Design review of the part built by this model. Coordinates are the model's own, in mm. A direction names the side the tool comes from. Round coordinates to 2 decimals unless told otherwise and drop trailing zeros. Write each loop counter-clockwise with the first axis right and the second up, starting at its lowest first coordinate (ties: lowest second). Pieces come first, ordered by that corner, then holes. Notation, with made-up numbers: (-19.5, -24.75) -> (-14.5, -24.75) arc R25 ccw to (-14.5, 11.25) -> close; hole circle Ø9 at (-25.5, 69.5). An arc over 180 degrees is marked (long way). One line per question, with ' | ' between items. Start each with the question number.
1) For probe 1 along Z at (x, y) = (-24.5, -16); probe 2 along Y at (x, z) = (-1.5, 101); probe 3 along Y at (x, z) = (-5.5, 125.5), list the stretches that pass through material, from the lowest coordinate up.
2) Insertion check: pin 1 Ø3.5 at (y, z) = (24, -1) entering from -X; pin 2 Ø18.5 at (x, y) = (3, -16.5) entering from +Z; pin 3 Ø8 at (x, z) = (-14, 12) entering from +Y; pin 4 Ø1.5 at (x, z) = (12.5, 80) entering from -Y. Each pin has a flat end and moves straight along its axis. Give the tip position at first contact, or say it passes through.
3) Consider section A-A (y = 0). Give the boundary of the cut face in (x, z) (3 decimals), then the cut area to 3 significant figures.
4) For faces 4 (the flat face through (6, 47.625, 64)), 5 (the flat face through (14.617, -24, -2)), 6 (the flat face through (6, 41.207, 66)), list the 3-axis set-ups (+Z, -Z, +X, -X, +Y, -Y) from which the entire face can be reached by the end or side of a thin tool; tool diameter is ignored.
5) Consider section C-C (x = 8). Give the boundary of the cut face in (y, z) (3 decimals), then the cut area to 3 significant figures.
6) Mouldability with a two-part tool opening along Y and no side actions: class faces 1 (the flat face through (17.792, 24, -2)), 2 (the flat face through (20.955, -1, -2)), 3 (the cylindrical face through (16.16, -39.688, -1.628)) as +Y half, -Y half, draft (parallel to the pull), parting line (faces both ways), or undercut.
7) Consider section D-D (y = -31.5). Give the boundary of the cut face in (x, z) (3 decimals), then the cut area to 3 significant figures.
8) Consider section B-B (z = 67). Give the boundary of the cut face in (x, y) (3 decimals).
```python
from build123d import *

# Parameters (mm, degrees)
F1_DEPTH = 133.35
F2_W     = 11.43
F2_H     = 95.25
F3_DEPTH = 6.35
F4_W     = 3.175
F4_H     = 7.62
F5_DEPTH = 3.302


with BuildPart() as f1:
    # F0 (on Top) → F1 (new body)
    with BuildSketch(Plane.XY):
        with BuildLine():
            Line((11.43, 47.625), (0, 47.625))
            ThreePointArc((0, 47.625), (-47.625, 0), (0, -47.625))
            Line((0, -47.625), (11.43, -47.625))
            Line((11.43, -47.625), (11.43, -41.232052))
            Line((11.43, -41.232052), (0, -41.232052))
            Line((0, -41.232052), (0, -41.275))
            ThreePointArc((0, -41.275), (-41.275, 0), (0, 41.275))
            Line((0, 41.275), (0, 41.207306))
            Line((0, 41.207306), (11.43, 41.207306))
            Line((11.43, 41.207306), (11.43, 47.625))
        make_face()
    extrude(amount=F1_DEPTH)

    # F2 (on Top) → F3 (join)
    with BuildSketch(Plane.XY):
        with BuildLine():
            Line((0, -47.625), (0, 47.625))
            ThreePointArc((0, 47.625), (-47.625, 0), (0, -47.625))
        make_face()
        with Locations((5.715, 0)):
            Rectangle(F2_W, F2_H)
    extrude(amount=-F3_DEPTH)

    # F4 (on face) → F5 (join)
    with BuildSketch(Plane.XY):
        with BuildLine():
            ThreePointArc((20.955, 38.890978), (16.227114, 39.752791), (11.43, 40.04145))
            Line((11.43, 40.04145), (11.43, -39.96855))
            ThreePointArc((11.43, -39.96855), (16.227114, -39.679891), (20.955, -38.818079))
            Line((20.955, -38.818079), (20.955, 38.890978))
        make_face()
        with Locations((16.204277, -24.09355)):
            Rectangle(F4_W, F4_H, mode=Mode.SUBTRACT)
        with Locations((16.1925, 0.03645)):
            Rectangle(F4_W, F4_H, mode=Mode.SUBTRACT)
        with Locations((16.204277, 24.16645)):
            Rectangle(F4_W, F4_H, mode=Mode.SUBTRACT)
    extrude(amount=-F5_DEPTH)


solid = f1.part
```
From the geometry:
1) probe 1: z = -6.35 to 0 | probe 2: y = -47.6 to -41.25, 41.25 to 47.6 | probe 3: y = -47.31 to -40.91, 40.91 to 47.31
2) pin 1: stops at x = -42.11 | pin 2: stops at z = 0 | pin 3: stops at y = 46.56 | pin 4: passes through
3) outline: (-47.625, -6.35) -> (11.43, -6.35) -> (11.43, -3.302) -> (14.605, -3.302) -> (14.605, 0) -> (-41.275, 0) -> (-41.275, 133.35) -> (-47.625, 133.35) -> close; (17.78, -3.302) -> (20.955, -3.302) -> (20.955, 0) -> (17.78, 0) -> close | area: 1,240 mm2
4) face 4: +Z, -Z, +X, -X, +Y | face 5: +Z, -Z | face 6: +Z, +X
5) outline: (-47.625, -6.35) -> (47.625, -6.35) -> (47.625, 133.35) -> (41.207, 133.35) -> (41.207, 0) -> (-41.232, 0) -> (-41.232, 133.35) -> (-47.625, 133.35) -> close | area: 2,310 mm2
6) face 1: undercut | face 2: draft | face 3: -Y half
7) outline: (-35.72, -6.35) -> (11.43, -6.35) -> (11.43, -3.302) -> (20.955, -3.302) -> (20.955, 0) -> (-26.672, 0) -> (-26.672, 133.35) -> (-35.72, 133.35) -> close | area: 1,540 mm2
8) outline: (0, -47.625) -> (11.43, -47.625) -> (11.43, -41.232) -> (0, -41.232) -> (0, -41.275) arc R41.275 cw to (0, 41.275) -> (0, 41.207) -> (11.43, 41.207) -> (11.43, 47.625) -> (0, 47.625) arc R47.625 ccw to start
